from build123d import *

# Parameters (mm, degrees)
F0_W     = 50
F0_H     = 50
F1_DEPTH = 3
F2_W     = 25
F2_H     = 25
F3_ANGLE = 20
F4_DEPTH = 6
F5_W     = 50
F5_H     = 50
F6_DEPTH = 3
F7_R     = 5
F8_R     = 5


with BuildPart() as f1:
    # F0 (on Top) → F1 (new body)
    with BuildSketch(Plane.XY):
        Rectangle(F0_W, F0_H)
    extrude(amount=F1_DEPTH)

    # F2 (on face) → F3 (revolve)
    with BuildSketch(Plane.XY.offset(3)):
        Rectangle(F2_W, F2_H)
    revolve(axis=Axis((0, -12.5, 3), (1, 0, 0)), revolution_arc=F3_ANGLE)

    # F4 (add): a face of the model
    f4_faces = [f1.faces().sort_by_distance(p)[0] for p in [
        (0, -0.7538422402, 7.2752517916),
    ]]
    extrude(f4_faces, amount=F4_DEPTH)

    # F5 (on face) → F6 (join)
    with BuildSketch(Plane(origin=(0, -4.478524505, 12.3046449499), x_dir=(1, 0, 0), z_dir=(0, -0.3420201433, 0.9396926208))):
        with Locations((0, 2.1972288873)):
            Rectangle(F5_W, F5_H)
    extrude(amount=F6_DEPTH)

    # F7
    f7_edges = [f1.edges().sort_by_distance(p)[0] for p in [
        (25, 20.565481, 23.016184),
        (-25, 20.565481, 23.016184),
        (-25, -26.41915, 5.915177),
        (25, -26.41915, 5.915177),
        (25, -25, 1.5),
        (-25, -25, 1.5),
        (-25, 25, 1.5),
        (25, 25, 1.5),
    ]]
    fillet(f7_edges, radius=F7_R)

    # F8
    f8_edges = [f1.edges().sort_by_distance(p)[0] for p in [
        (12.5, 9.966255, 14.369581),
        (-12.5, 9.966255, 14.369581),
        (-12.5, -13.52606, 5.819078),
        (12.5, -13.52606, 5.819078),
    ]]
    fillet(f8_edges, radius=F8_R)


solid = f1.part
For this review, take the finished solid that the model builds, in its own axes (mm). A direction names the side the tool comes from. Round coordinates to 2 decimals unless told otherwise and drop trailing zeros. Order: outer loops, then holes, each group sorted by start corner. A loop starts at its lowest first (then second) coordinate and runs counter-clockwise, first axis right, second up. Notation, with made-up numbers: (44.5, 36.5) -> (102.5, 36.5) arc R5 cw to (102.5, 40.5) -> close; hole circle Ø4 at (36.5, -21). An arc over 180 degrees is marked (long way). Write item = value, one per line. Start each with the question number.
1) Take a section at C-C on y = 14. State the section outline as (x, z) points, plus the area to 3 significant figures.
2) To check wall thickness, follow line 1 (Z direction, x = 16, y = -5); line 2 (Z direction, x = 17.5, y = -13); line 3 (Z direction, x = -8, y = -4.5). State the ranges of each line that lie inside material, in increasing order. Write a range as from..to.
3) Take a section at A-A on x = -15. State the section outline as (y, z) points.
4) Insertion check: pin 1 (1.5 mm diameter, centred on x = -19, z = 2.5, fed in from -Y); pin 2 (1.5 mm diameter, centred on x = -6.5, z = 8, fed in from +Y); pin 3 (15 mm diameter, centred on x = 0.5, y = -9, fed in from +Z). Each pin has a flat end and moves straight along its axis. Give the tip position at first contact, or say it passes through.
5) Tool access review of faces 1 (the face through (12.5, -1, 8)), 2 (the face through (10.761, 8.356, 16.976)), 3 (the face through (0.11, 12.13, 7.28)): name each direction out of +Z, -Z, +X, -X, +Y, -Y from which nothing blocks a thin tool from reaching the whole face with its end or side.
6) The part is to be moulded in two halves that separate along Z. For faces 4 (the face through (-23.57, 19.15, 22.52)), 5 (the face through (-12.5, -1, 8)), 6 (the face through (-24, -23, 2)), say which applies: +Z half, -Z half, draft (parallel to the pull), parting line (faces both ways), or undercut.
7) Take a section at B-B on x = 6. State the section outline as (y, z) points.
Verdict:
q1.outline = (-25, 0) -> (25, 0) -> (25, 3) -> (-25, 3) -> close; (-25, 19.03) -> (25, 19.03) -> (25, 22.22) -> (-25, 22.22) -> close
q1.area = 310 mm2
q2.line_1 = 0..3, 12.11..15.31
q2.line_2 = 0..3, 9.2..12.4
q2.line_3 = 0..15.49
q3.outline = (-26.93, 7.32) -> (-25.91, 4.51) -> (21.08, 21.61) -> (20.05, 24.43) -> close; (-25, 0) -> (25, 0) -> (25, 3) -> (-25, 3) -> close
q4.pin_1 = -25
q4.pin_2 = 12.14
q4.pin_3 = 16.58
q5.face_1 = +X, +Y
q5.face_2 = none
q5.face_3 = +X, -X, +Y
q6.face_4 = +Z half
q6.face_5 = undercut
q6.face_6 = draft
q7.outline = (-26.93, 7.32) -> (-25.91, 4.51) -> (-14.55, 8.64) -> (-12.5, 3) -> (-25, 3) -> (-25, 0) -> (25, 0) -> (25, 3) -> (12.5, 3) arc R25 ccw to (10.99, 11.55) -> (8.94, 17.19) -> (21.08, 21.61) -> (20.05, 24.43) -> close
